```python
from build123d import *

# Parameters (mm, degrees)
ESQUISSE1_W        = 15
ESQUISSE1_H        = 50
BOSS_EXTRU_1_DEPTH = 15
CONG_1_R           = 20


with BuildPart() as part:
    # Esquisse1 → Boss.-Extru.1 (new body)
    with BuildSketch(Plane.XY):
        Polygon((0, 0), (55, 0), (55, 110), (70, 110), (70, 0), (125, 0), (125, 800), (0, 800), align=None)
        with Locations((62.5, 185)):
            Rectangle(ESQUISSE1_W, ESQUISSE1_H, mode=Mode.SUBTRACT)
        with Locations((62.5, 285)):
            Rectangle(ESQUISSE1_W, ESQUISSE1_H, mode=Mode.SUBTRACT)
        with Locations((62.5, 385)):
            Rectangle(ESQUISSE1_W, ESQUISSE1_H, mode=Mode.SUBTRACT)
        with Locations((62.5, 485)):
            Rectangle(ESQUISSE1_W, ESQUISSE1_H, mode=Mode.SUBTRACT)
        with Locations((62.5, 585)):
            Rectangle(ESQUISSE1_W, ESQUISSE1_H, mode=Mode.SUBTRACT)
        with Locations((62.5, 685)):
            Rectangle(ESQUISSE1_W, ESQUISSE1_H, mode=Mode.SUBTRACT)
    extrude(amount=BOSS_EXTRU_1_DEPTH)

    # Congé1
    cong_1_edges = [part.edges().sort_by_distance(p)[0] for p in [
        (0, 800, 7.5),
        (125, 800, 7.5),
        (125, 0, 7.5),
        (70, 0, 7.5),
        (55, 0, 7.5),
        (0, 0, 7.5),
    ]]
    fillet(cong_1_edges, radius=CONG_1_R)


solid = part.part
```
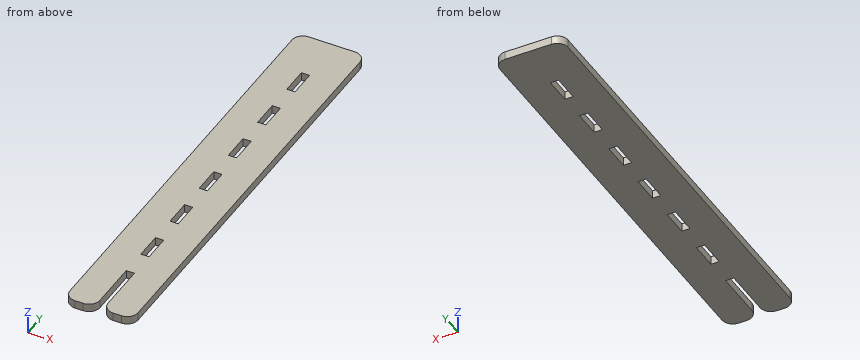
CAD build for the part. Positions are in the model's coordinates, mm. Give positions to 0.01 mm unless a question says otherwise; leave off trailing zeros. Loops run counter-clockwise (first coordinate to the right, second up) from the corner with the lowest first, then second, coordinate; pieces in that order, holes last. Notation, with made-up numbers: (14, 47.5) - (18, 47.5) arc R19 cw to (18, 66.5) - close; hole circle Ø10 at (-27.75, 74.5). An arc over 180 degrees is marked (long way). Put each result on its own line as item: value.
Q1. Flat gauge pins, fed straight in: pin 1 (10 mm diameter, centred on x = 95, y = 636, fed in from -Z); pin 2 (4 mm diameter, centred on x = 50.5, z = 12.5, fed in from -Y); pin 3 (4.5 mm diameter, centred on x = 64.5, z = 9, fed in from -Y). Where does each tip first touch, or does it go through?
Filled in:
pin 1: stops at z = 0
pin 2: stops at y = 5.24
pin 3: stops at y = 110
Q2. Slice it at A-A (y = 266.5). Give the cut face in (x, z), plus the area to 3 significant figures.
Filled in:
outline: (0, 0) - (55, 0) - (55, 15) - (0, 15) - close; (70, 0) - (125, 0) - (125, 15) - (70, 15) - close
area: 1,650 mm²
Q3. Probe line 1 along X through (y, z) = (62, 13); line 2 along Y through (x, z) = (109, 13.5); line 3 along Y through (x, z) = (42, 1) (3 decimals). List the from-to ranges inside material, lowest first.
Filled in:
line 1: x = 0 to 55, 70 to 125
line 2: y = 0.4 to 799.6
line 3: y = 1.265 to 800
Q4. Slice it at B-B (z = 3). Give the number of separate pieces and of enclosed holes in the cut face, plus the area to 3 significant figures.
Filled in:
separate pieces: 1
enclosed holes: 6
area: 93,300 mm²
